For this review, take the finished solid that the model builds, in its own axes (mm). A direction names the side the tool comes from. Coordinates: 2 decimals unless noted, no trailing zeros. Loops run counter-clockwise (first coordinate to the right, second up) from the corner with the lowest first, then second, coordinate; pieces in that order, holes last. Notation, with made-up numbers: M -10.75,81 L 29.25,81 A22 ccw 29.25,89 Z; hole C 83,42 d3. An arc over 180 degrees is marked long. Answer as a JSON object with one key per item and string values. Group by question number.
Item 1: Mouldability with a two-part tool opening along X and no side actions: class faces 1 (the face through (74.421, 1, -22)), 2 (the face through (26, 1, 16.51)), 3 (the face through (2.6, 1, -7)) as +X half, -X half, draft (parallel to the pull), parting line (faces both ways), or undercut.
Item 2: Tool access review of faces 4 (the face through (53.276, 1, -54)), 5 (the face through (-1.65, 1, -25)), 6 (the face through (63, 1, -48.8)): name each direction out of +Z, -Z, +X, -X, +Y, -Y from which nothing blocks a thin tool from reaching the whole face with its end or side.
Item 3: Add section A-A (x = 4). State the section outline as (y, z) points.
Item 4: Add section D-D (x = 29.5). State the section outline as (y, z) points, then the cut area to 3 significant figures.
Item 5: Add section B-B (y = 1.6). State the section outline as (x, z) points.
Item 6: Add section C-C (z = 0.5). State the section outline as (x, y) points, then the cut area to 3 significant figures.
Item 7: Insertion check: pin 1 (1.5 mm diameter, centred on x = 49.5, y = 1.5, fed in from -Z); pin 2 (1 mm diameter, centred on y = 2.5, z = 8, fed in from +X); pin 3 (1.8 mm diameter, centred on x = -3.302, z = -52.324, fed in from +Y); pin 4 (1.5 mm diameter, centred on x = 62, y = 2, fed in from +Z). Each pin has a flat end and moves straight along its axis. Give the tip position at first contact, or say it passes through.
Item 8: Wall thickness on L1, parallel to X at y = 0.95, z = -5.08; L2, parallel to Z at x = 4.5, y = 2.1; L3, parallel to X at y = 1.7, z = -29.5: over which ranges is each line inside the solid? List them lowest first. Write a range as from..to.
from build123d import *

# Parameters (mm, degrees)
SKETCH_1_R      = 1.5
SKETCH_1_W      = 6.3
SKETCH_1_H      = 5
SKETCH_1_W_2    = 27
SKETCH_1_H_2    = 27
EXTRUDE_1_DEPTH = 3
CHAMFER_1_SIZE  = 1


with BuildPart() as part:
    # 草图1 → 凸台-拉伸1 (new body)
    with BuildSketch(Plane(origin=(0, 0, 0), x_dir=(1, 0, 0), z_dir=(0, 1, 0))):
        Polygon((-7.176, 56.452), (-7.176, -16.51), (60.7, -16.51), (60.7, 12), (74.421, 12), (74.421, 32.5), (52.8, 32.5), (52.8, 48.8), (74.421, 48.8), (74.421, 56.452), (53.276, 56.452), (53.276, 50.8), (2.6, 50.8), (2.6, 56.452), align=None)
        with Locations(Location((-3.302, -12.192, 0), (0, 0, 270))):
            Circle(SKETCH_1_R, mode=Mode.SUBTRACT)
        with Locations((-0.55, 7.5)):
            Rectangle(SKETCH_1_W, SKETCH_1_H, mode=Mode.SUBTRACT)
        with Locations(Location((57.404, 5.08, 0), (0, 0, 270))):
            Circle(SKETCH_1_R, mode=Mode.SUBTRACT)
        with Locations((11.85, 24.75)):
            Rectangle(SKETCH_1_W_2, SKETCH_1_H_2, mode=Mode.SUBTRACT)
        with Locations(Location((-3.302, 52.324, 0), (0, 0, 270))):
            Circle(SKETCH_1_R, mode=Mode.SUBTRACT)
        with Locations(Location((56.388, 53.34, 0), (0, 0, 270))):
            Circle(SKETCH_1_R, mode=Mode.SUBTRACT)
    extrude(amount=EXTRUDE_1_DEPTH)

    # 倒角1
    chamfer_1_edges = [part.edges().sort_by_distance(p)[0] for p in [
        (53.276, 1.5, -50.8),
    ]]
    chamfer(chamfer_1_edges, length=CHAMFER_1_SIZE)


solid = part.part
From the geometry:
{
 "1": {"face 1": "+X half", "face 2": "draft", "face 3": "undercut"},
 "2": {"face 4": "-Z, +Y, -Y", "face 5": "+Y, -Y", "face 6": "+X, +Y, -Y"},
 "3": {"outline": "M 0,-50.8 L 3,-50.8 L 3,-38.25 L 0,-38.25 Z; M 0,-11.25 L 3,-11.25 L 3,16.51 L 0,16.51 Z"},
 "4": {"outline": "M 0,-50.8 L 3,-50.8 L 3,16.51 L 0,16.51 Z", "area": "202 mm²"},
 "5": {"outline": "M -7.18,-56.45 L 2.6,-56.45 L 2.6,-50.8 L 52.28,-50.8 L 53.28,-51.8 L 53.28,-56.45 L 74.42,-56.45 L 74.42,-48.8 L 52.8,-48.8 L 52.8,-32.5 L 74.42,-32.5 L 74.42,-12 L 60.7,-12 L 60.7,16.51 L -7.18,16.51 Z; hole C -3.3,-52.32 d3; hole C -3.3,12.19 d3; hole M -3.7,-10 L 2.6,-10 L 2.6,-5 L -3.7,-5 Z; hole M -1.65,-38.25 L 25.35,-38.25 L 25.35,-11.25 L -1.65,-11.25 Z; hole C 56.39,-53.34 d3; hole C 57.4,-5.08 d3"},
 "6": {"outline": "M -7.18,0 L 60.7,0 L 60.7,3 L -7.18,3 Z", "area": "204 mm²"},
 "7": {"pin 1": "stops at z = -50.8", "pin 2": "stops at x = 60.7", "pin 3": "passes through", "pin 4": "stops at z = -12"},
 "8": {"L1": "x = -7.18..-3.7, 2.6..55.9, 58.9..60.7", "L2": "z = -50.8..-38.25, -11.25..16.51", "L3": "x = -7.18..-1.65, 25.35..74.42"}
}
